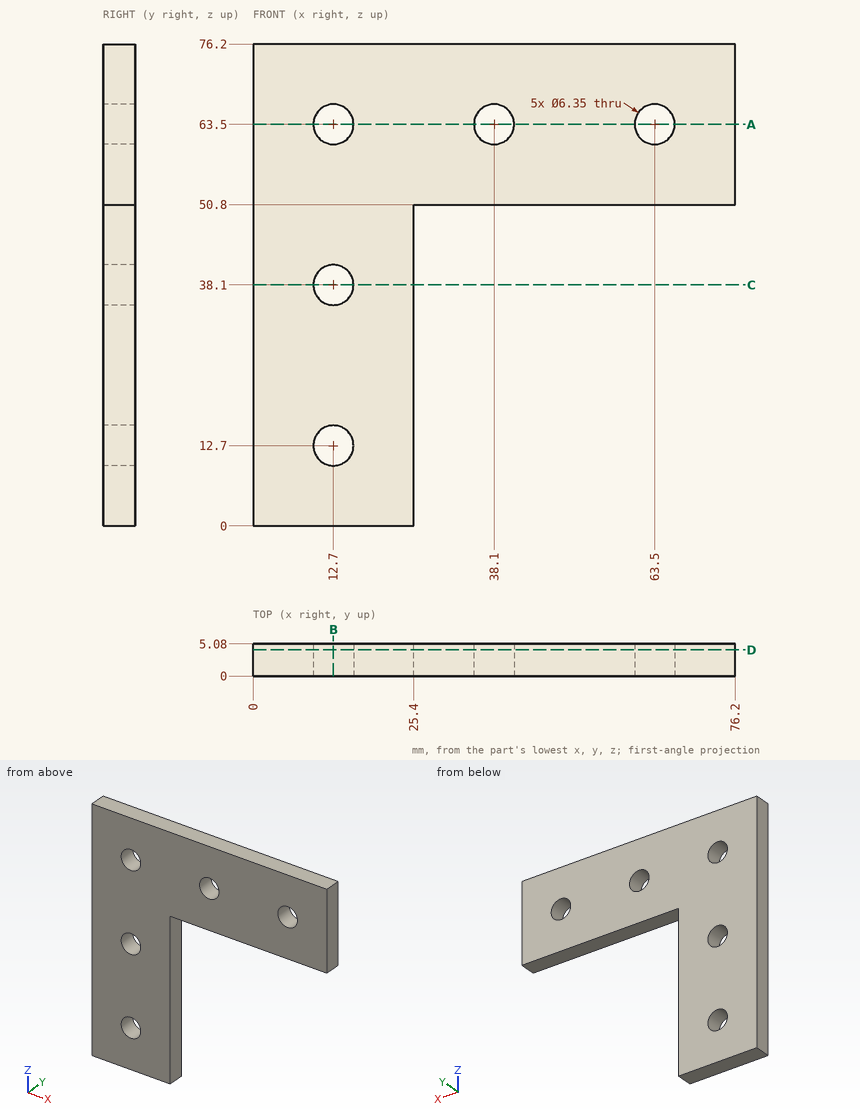
Part print with two shaded views. Sizes in mm from the minimum x, y, z corner. Round coordinates to 2 decimals unless told otherwise and drop trailing zeros. Order: outer loops, then holes, each group sorted by start corner. A loop starts at its lowest first (then second) coordinate and runs counter-clockwise, first axis right, second up. Notation, with made-up numbers: (33, 30) - (43, 30) arc R20 cw to (43, 55) - close; hole circle Ø4 at (67, 76.5). An arc over 180 degrees is marked (long way). Return JSON: item names as keys, results as strings.
(1) Cut at C-C (z = 38.1). Give the cut face in (x, y) (3 decimals).
Answer key:
{"outline": "(0, 0) - (9.525, 0) - (9.525, 5.08) - (0, 5.08) - close; (15.875, 0) - (25.4, 0) - (25.4, 5.08) - (15.875, 5.08) - close"}
(2) Wall check: probe 1 along X at (y, z) = (3.6, 63.5) (3 decimals); probe 2 along Z at (x, y) = (14, 0.25). Give the ranges that are in metal, low to high. Write a range as from..to.
Answer key:
{"probe 1": "x = 0..9.525, 15.875..34.925, 41.275..60.325, 66.675..76.2", "probe 2": "z = 0..9.8, 15.6..35.2, 41..60.6, 66.4..76.2"}
(3) Cut at D-D (y = 4.15). Give the cut face in (x, z) (3 decimals), then the cut area to 3 significant figures.
Answer key:
{"outline": "(0, 0) - (25.4, 0) - (25.4, 50.8) - (76.2, 50.8) - (76.2, 76.2) - (0, 76.2) - close; hole circle Ø6.35 at (12.7, 12.7); hole circle Ø6.35 at (12.7, 38.1); hole circle Ø6.35 at (12.7, 63.5); hole circle Ø6.35 at (38.1, 63.5); hole circle Ø6.35 at (63.5, 63.5)", "area": "3,070 mm^2"}
(4) Pin check, flat tips, straight feed: pin 1 Ø4 at (x, z) = (38.1, 63.5) entering from +Y; pin 2 Ø2.5 at (y, z) = (2, 38) entering from +X; pin 3 Ø3 at (x, y) = (35.5, 1) entering from -Z. Stop position of each tip, or through.
Answer key:
{"pin 1": "passes through", "pin 2": "stops at x = 25.4", "pin 3": "stops at z = 50.8"}
(5) Cut at B-B (x = 12.7). Give the cut face in (y, z) (3 decimals), then the cut area to 3 significant figures.
Answer key:
{"outline": "(0, 0) - (5.08, 0) - (5.08, 9.525) - (0, 9.525) - close; (0, 15.875) - (5.08, 15.875) - (5.08, 34.925) - (0, 34.925) - close; (0, 41.275) - (5.08, 41.275) - (5.08, 60.325) - (0, 60.325) - close; (0, 66.675) - (5.08, 66.675) - (5.08, 76.2) - (0, 76.2) - close", "area": "290 mm^2"}
(6) Cut at A-A (z = 63.5). Give the cut face in (x, y) (3 decimals).
Answer key:
{"outline": "(0, 0) - (9.525, 0) - (9.525, 5.08) - (0, 5.08) - close; (15.875, 0) - (34.925, 0) - (34.925, 5.08) - (15.875, 5.08) - close; (41.275, 0) - (60.325, 0) - (60.325, 5.08) - (41.275, 5.08) - close; (66.675, 0) - (76.2, 0) - (76.2, 5.08) - (66.675, 5.08) - close"}
